Can you work these out from the model? Positions are in its coordinate system, mm. A direction names the side the tool comes from. Give positions to 0.01 mm unless a question says otherwise; leave off trailing zeros. Order: outer loops, then holes, each group sorted by start corner. A loop starts at its lowest first (then second) coordinate and runs counter-clockwise, first axis right, second up. Notation, with made-up numbers: (55, -24.75) - (109, -24.75) arc R22 cw to (109, -2.75) - close; hole circle Ø10 at (13, 33.5). An arc over 180 degrees is marked (long way). Use one line per item in the form item = value. Start each with the question number.
1) Which directions (+Z, -Z, +X, -X, +Y, -Y) give clear straight access to the entire face, cutting with the end or side of a thin tool? Please do faces 4 (the flat face through (-24, 12, -17.5)), 5 (the flat face through (-22.5, 7, 0)), 6 (the flat face through (23, 4.3, 0)), 7 (the flat face through (3, 10.507, 26)).
2) Suppose I cut it at A-A, the plane y = 5. Write out the boundary of the cut face in (x, z), and give its area (3 significant figures).
3) For pin 1 (4 mm diameter, centred on x = -9.5, z = 18.5, fed in from +Y); pin 2 (0.6 mm diameter, centred on x = -23.5, z = -4, fed in from +Y); pin 3 (2 mm diameter, centred on x = -24, z = 0, fed in from +Y), each with a flat end and sliding along its axis, tell me the tip position at first contact or that it passes through.
4) We'd pull the mould along X, two halves only. Please class faces 1 (the flat face through (0, 7, -25)), 2 (the flat face through (-24, 12, 1.5)), 3 (the cylindrical face through (-2.243, 11.218, 26.014)): released by +X, released by -X, zero draft, split by the parting line, or undercut.
5) Suppose I cut it at C-C, the plane x = 11. Write out the boundary of the cut face in (y, z), and give its area (3 significant figures).
6) Please list where these lines run through material, in increasing order: probe 1 along X at (y, z) = (7.5, -20); probe 2 along Z at (x, y) = (21, 2.5); probe 3 along Z at (x, y) = (-10, 5).
7) Suppose I cut it at B-B, the plane z = -4. Write out the boundary of the cut face in (x, y).
```python
from build123d import *

# Parameters (mm, degrees)
SKETCH1_W             = 49
SKETCH1_H             = 54
BOSS_EXTRUDE1_DEPTH   = 2
SKETCH2_W             = 49
SKETCH2_H             = 54
SKETCH2_W_2           = 45
SKETCH2_H_2           = 50
EXTRUDE_THIN1_DEPTH   = 11
SKETCH7_W             = 6
SKETCH7_H             = 2
CUT_EXTRUDE1_DEPTH    = 2
SKETCH6_W             = 12
SKETCH6_H             = 2
CUT_EXTRUDE2_DEPTH    = 2
CUT_EXTRUDE3_DEPTH    = 2
SKETCH15_R            = 1.75
BOSS_EXTRUDE2_DEPTH   = 11
BOSS_EXTRUDE2_2_DEPTH = 11
BOSS_EXTRUDE2_3_DEPTH = 11
BOSS_EXTRUDE2_4_DEPTH = 11
SKETCH17_R            = 0.9
BOSS_EXTRUDE3_DEPTH   = 15
CUT_EXTRUDE4_DEPTH    = 49
FILLET1_R             = 1


with BuildPart() as part:
    # Sketch1 → Boss-Extrude1 (new body)
    with BuildSketch(Plane(origin=(0, 0, 0), x_dir=(1, 0, 0), z_dir=(0, 1, 0))):
        Rectangle(SKETCH1_W, SKETCH1_H)
    extrude(amount=BOSS_EXTRUDE1_DEPTH)

    # Sketch2 → Extrude-Thin1 (add)
    with BuildSketch(Plane(origin=(0, 2, 0), x_dir=(1, 0, 0), z_dir=(0, 1, 0))):
        Rectangle(SKETCH2_W, SKETCH2_H)
        Rectangle(SKETCH2_W_2, SKETCH2_H_2, mode=Mode.SUBTRACT)
    extrude(amount=EXTRUDE_THIN1_DEPTH)

    # Sketch7 → Cut-Extrude1 (cut)
    with BuildSketch(Plane.ZY.offset(24.5)):
        with Locations((-4.5, 12)):
            Rectangle(SKETCH7_W, SKETCH7_H)
        with Locations((-14.5, 12)):
            Rectangle(SKETCH7_W, SKETCH7_H)
    extrude(amount=-CUT_EXTRUDE1_DEPTH, mode=Mode.SUBTRACT)

    # Sketch6 → Cut-Extrude2 (cut)
    with BuildSketch(Plane.ZY.offset(24.5)):
        with Locations((7.5, 12)):
            Rectangle(SKETCH6_W, SKETCH6_H)
    extrude(amount=-CUT_EXTRUDE2_DEPTH, mode=Mode.SUBTRACT)

    # Sketch14 → Cut-Extrude3 (cut)
    with BuildSketch(Plane.XY.offset(27)):
        with BuildLine():
            Line((-0.5, 15.493238672), (5.5, 15.493238672))
            ThreePointArc((5.5, 15.493238672), (7.993238672, 13), (5.5, 10.506761328))
            Line((5.5, 10.506761328), (-0.5, 10.506761328))
            ThreePointArc((-0.5, 10.506761328), (-2.993238672, 13), (-0.5, 15.493238672))
        make_face()
    extrude(amount=-CUT_EXTRUDE3_DEPTH, mode=Mode.SUBTRACT)



with BuildPart() as body_2:
    # Sketch15 → Boss-Extrude2 (new body)
    with BuildSketch(Plane(origin=(0, 2, 0), x_dir=(1, 0, 0), z_dir=(0, 1, 0))):
        with Locations((-22.5, -25)):
            Circle(SKETCH15_R)
    extrude(amount=BOSS_EXTRUDE2_DEPTH)


with BuildPart() as body_3:
    # Sketch15 → Boss-Extrude2 2 (new body)
    with BuildSketch(Plane(origin=(0, 2, 0), x_dir=(1, 0, 0), z_dir=(0, 1, 0))):
        with Locations((-22.5, 25)):
            Circle(SKETCH15_R)
    extrude(amount=BOSS_EXTRUDE2_2_DEPTH)


with BuildPart() as body_4:
    # Sketch15 → Boss-Extrude2 3 (new body)
    with BuildSketch(Plane(origin=(0, 2, 0), x_dir=(1, 0, 0), z_dir=(0, 1, 0))):
        with Locations((22.5, 25)):
            Circle(SKETCH15_R)
    extrude(amount=BOSS_EXTRUDE2_3_DEPTH)


with BuildPart() as body_5:
    # Sketch15 → Boss-Extrude2 4 (new body)
    with BuildSketch(Plane(origin=(0, 2, 0), x_dir=(1, 0, 0), z_dir=(0, 1, 0))):
        with Locations((22.5, -25)):
            Circle(SKETCH15_R)
    extrude(amount=BOSS_EXTRUDE2_4_DEPTH)


with BuildPart() as part_1:
    add(part.part)

    add(body_2.part)  # Boss-Extrude3 merges body 2

    add(body_3.part)  # Boss-Extrude3 merges body 3

    add(body_4.part)  # Boss-Extrude3 merges body 4

    add(body_5.part)  # Boss-Extrude3 merges body 5
    # Sketch17 → Boss-Extrude3 (add)
    with BuildSketch(Plane(origin=(0, 2, 0), x_dir=(1, 0, 0), z_dir=(0, 1, 0))):
        with Locations((-22.5, -25)):
            Circle(SKETCH17_R)
        with Locations((22.5, -25)):
            Circle(SKETCH17_R)
        with Locations((22.5, 25)):
            Circle(SKETCH17_R)
        with Locations((-22.5, 25)):
            Circle(SKETCH17_R)
    extrude(amount=BOSS_EXTRUDE3_DEPTH)

    # Sketch21 → Cut-Extrude4 (cut)
    with BuildSketch(Plane.ZY.offset(24.5)):
        Polygon((0, 2.5), (-13, 2.5), (-13, 4.3), (13, 4.3), (13, 2.5), align=None)
    extrude(amount=-CUT_EXTRUDE4_DEPTH, mode=Mode.SUBTRACT)

    # Fillet1
    fillet1_edges = [part_1.edges().sort_by_distance(p)[0] for p in [
        (-24.5, 6.5, -27),
        (24.5, 6.5, -27),
        (24.5, 6.5, 27),
        (-24.5, 6.5, 27),
    ]]
    fillet(fillet1_edges, radius=FILLET1_R)


solid = part_1.part
```
Result sheet:
q1.face_4 = -X, +Y
q1.face_5 = +Y
q1.face_6 = +X, -X
q1.face_7 = +Z, +Y
q2.outline = (-24.5, -26) arc R1 ccw to (-23.5, -27) - (23.5, -27) arc R1 ccw to (24.5, -26) - (24.5, 26) arc R1 ccw to (23.5, 27) - (-23.5, 27) arc R1 ccw to (-24.5, 26) - close; hole (-22.5, -23.25) arc R1.75 cw to (-20.75, -25) - (20.75, -25) arc R1.75 cw to (22.5, -23.25) - (22.5, 23.25) arc R1.75 cw to (20.75, 25) - (-20.75, 25) arc R1.75 cw to (-22.5, 23.25) - close
q2.area = 405 mm²
q3.pin_1 = 2
q3.pin_2 = 11
q3.pin_3 = 13
q4.face_1 = undercut
q4.face_2 = zero draft
q4.face_3 = undercut
q5.outline = (0, -27) - (13, -27) - (13, -25) - (2, -25) - (2, 25) - (13, 25) - (13, 27) - (0, 27) - close
q5.area = 152 mm²
q6.probe_1 = -24.5 to -22.5, 22.5 to 24.5
q6.probe_2 = -27 to -24.1, 24.1 to 27
q6.probe_3 = -27 to -25, 25 to 27
q7.outline = (-24.5, 0) - (24.5, 0) - (24.5, 2.5) - (22.5, 2.5) - (22.5, 2) - (-22.5, 2) - (-22.5, 2.5) - (-24.5, 2.5) - close; (-24.5, 4.3) - (-22.5, 4.3) - (-22.5, 11) - (-24.5, 11) - close; (22.5, 4.3) - (24.5, 4.3) - (24.5, 13) - (22.5, 13) - close
